Design review of the part built by this model. Coordinates are the model's own, in mm. A direction names the side the tool comes from. Give positions to 0.01 mm unless a question says otherwise; leave off trailing zeros. Loops run counter-clockwise (first coordinate to the right, second up) from the corner with the lowest first, then second, coordinate; pieces in that order, holes last. Notation, with made-up numbers: (-13, -24.5) -> (23, -24.5) arc R31 cw to (23, 7.5) -> close; hole circle Ø1 at (17.5, 75). An arc over 180 degrees is marked (long way). Answer in a Markdown table with one row per item. Add a question column.
(1) Consider section D-D on y = 18.5. Write out the cut boundary in (x, z).
(2) Consider section A-A on x = 0. Write out the cut boundary in (y, z).
(3) Consider section B-B on z = 14.5. Write out the cut boundary in (x, y), then the cut area to 3 significant figures.
(4) Draft analysis for pull direction Z (two halves, no side actions). For faces 1 (the cylindrical face through (0.07, 1.48, 12.5)), 2 (the cylindrical face through (-6.834, 14.44, -1.517)), 3 (the flat face through (-4, 34, 0)), 4 (the cylindrical face through (-13.55, 1.48, 1.43)), state which applies: +Z half, -Z half, draft (parallel to the pull), parting line (faces both ways), or undercut.
(5) For line 1 (X direction, y = 1.95, z = 0); line 2 (Y direction, x = -9.5, z = 7); line 3 (Y direction, x = -4.5, z = 2), list the stretches that pass through material, from the lowest coordinate up.
(6) Consider section C-C on x = 14. Write out the cut boundary in (y, z).
(7) For pin 1 (3.5 mm diameter, centred on y = 33, z = 1, fed in from -X); pin 2 (4 mm diameter, centred on x = 0, z = 14, fed in from +Y); pin 3 (2.5 mm diameter, centred on x = -14, z = 0, fed in from +Y); pin 4 (4 mm diameter, centred on y = 16, z = -4.5, fed in from -X), all flat-tipped, find the tip position at first contact; note any pin that passes through.
(8) For faces 5 (the flat face through (-5, 26, 0)), 6 (the cylindrical face through (16.855, 1.479, -2.213)), list the 3-axis set-ups (+Z, -Z, +X, -X, +Y, -Y) from which the entire face can be reached by the end or side of a thin tool; tool diameter is ignored.
from build123d import *

# Parameters (mm, degrees)
SKETCH_1_R      = 17
SKETCH_1_R_2    = 1.5
EXTRUDE_1_DEPTH = 3
SKETCH_2_R      = 7
EXTRUDE_2_DEPTH = 23
EXTRUDE_3_DEPTH = 16.5
FILLET_1_R      = 0.2


with BuildPart() as part:
    # 草图1 → 凸台-拉伸1 (new body)
    with BuildSketch(Plane(origin=(0, 0, 0), x_dir=(1, 0, 0), z_dir=(0, 1, 0))):
        with Locations(Location((0, 0, 0), (0, 0, 270))):
            Circle(SKETCH_1_R)
        with Locations(Location((0, 14, 0), (0, 0, 270))):
            Circle(SKETCH_1_R_2, mode=Mode.SUBTRACT)
        with Locations(Location((14, 0, 0), (0, 0, 270))):
            Circle(SKETCH_1_R_2, mode=Mode.SUBTRACT)
        with Locations(Location((0, -14, 0), (0, 0, 270))):
            Circle(SKETCH_1_R_2, mode=Mode.SUBTRACT)
        with Locations(Location((-14, 0, 0), (0, 0, 270))):
            Circle(SKETCH_1_R_2, mode=Mode.SUBTRACT)
    extrude(amount=EXTRUDE_1_DEPTH)

    # 草图2 → 凸台-拉伸2 (add)
    with BuildSketch(Plane(origin=(0, 3, 0), x_dir=(1, 0, 0), z_dir=(0, 1, 0))):
        with Locations(Location((0, 0, 0), (0, 0, 270))):
            Circle(SKETCH_2_R)
    extrude(amount=EXTRUDE_2_DEPTH)

    # 草图3 → 凸台-拉伸3 (add)
    with BuildSketch(Plane(origin=(0, 26, 0), x_dir=(1, 0, 0), z_dir=(0, 1, 0))):
        with BuildLine():
            Line((-4, 0), (-4, 3))
            ThreePointArc((-4, 3), (5, 0), (-4, -3))
            Line((-4, -3), (-4, 0))
        make_face()
    extrude(amount=EXTRUDE_3_DEPTH)

    # 圆角1
    fillet_1_edges = [part.edges().sort_by_distance(p)[0] for p in [
        (0, 3, -7),
        (5, 26, 0),
        (5, 42.5, 0),
    ]]
    fillet(fillet_1_edges, radius=FILLET_1_R)


solid = part.part
Values follow:
| question | item | result |
|---|---|---|
| 1 | outline | circle Ø14 at (0, 0) |
| 2 | outline | (0, -17) -> (3, -17) -> (3, -15.5) -> (0, -15.5) -> close; (0, -12.5) -> (3, -12.5) -> (3, -7.2) arc R0.2 cw to (3.2, -7) -> (26, -7) -> (26, -5.2) arc R0.2 cw to (26.2, -5) -> (42.3, -5) arc R0.2 ccw to (42.5, -4.8) -> (42.5, 4.8) arc R0.2 ccw to (42.3, 5) -> (26.2, 5) arc R0.2 cw to (26, 5.2) -> (26, 7) -> (3.2, 7) arc R0.2 cw to (3, 7.2) -> (3, 12.5) -> (0, 12.5) -> close; (0, 15.5) -> (3, 15.5) -> (3, 17) -> (0, 17) -> close |
| 3 | outline | (-8.87, 0) -> (-1.41, 0) -> (-1.41, 3) -> (-8.87, 3) -> close; (1.41, 0) -> (8.87, 0) -> (8.87, 3) -> (1.41, 3) -> close |
| 3 | area | 44.8 mm2 |
| 4 | face 1 | undercut |
| 4 | face 2 | parting line |
| 4 | face 3 | draft |
| 4 | face 4 | undercut |
| 5 | line 1 | -17 to -15.5, -12.5 to 12.5, 15.5 to 17 |
| 5 | line 2 | 0 to 3 |
| 5 | line 3 | 0 to 26 |
| 6 | outline | (0, -9.64) -> (3, -9.64) -> (3, -1.5) -> (0, -1.5) -> close; (0, 1.5) -> (3, 1.5) -> (3, 9.64) -> (0, 9.64) -> close |
| 7 | pin 1 | x = -4 |
| 7 | pin 2 | y = 3 |
| 7 | pin 3 | through |
| 7 | pin 4 | x = -6.54 |
| 8 | face 5 | +Y |
| 8 | face 6 | +Y, -Y |
